Geometry: final body of the model. Coordinates: model frame, mm. A direction names the side the tool comes from. Give positions to 0.01 mm unless a question says otherwise; leave off trailing zeros. Write each loop counter-clockwise with the first axis right and the second up, starting at its lowest first coordinate (ties: lowest second). Pieces come first, ordered by that corner, then holes.
Q1. Draft query along Y for faces 6 (the face through (0, 31.828, 21)), 7 (the face through (-34, 13, -19.964)), 8 (the face through (34.03, 12.53, 21.44)). Return one class per face: pulls with the +Y half, pulls with the -Y half, needs draft (parallel to the pull), parting line crosses it, or undercut.
Q2. Cut plane D-D on y = 14.25. Return the cut outline in (x, z) (3 decimals), plus the area to 3 significant figures.
Q3. Line query: L1, parallel to Z at x = 30.5, y = 9.5; L2, parallel to Y at x = -23, z = -13; L3, parallel to Z at x = 23.5, y = 18. Output: solid intervals per line, ascending.
Q4. Pin query (flat end, axial travel): pin 1 (6.5 mm diameter, centred on y = 25, z = -16.5, fed in from +X) (3 decimals); pin 2 (6 mm diameter, centred on x = -25.5, y = 26, fed in from -Z); pin 3 (5 mm diameter, centred on x = -10.5, y = 24, fed in from -Z). Return the tip coordinate at first contact, or that it passes through.
Q5. Cut plane A-A on y = 22. Return the cut outline in (x, z) (1 decimal).
Q6. Cut plane B-B on z = 8. Return the cut outline in (x, y) (1 decimal).
Q7. Cut plane C-C on x = -3. Return the cut outline in (y, z).
Q8. Reachability of faces 1 (the face through (-4, 26.828, -15)), 2 (the face through (-1.495, 24.5, -15.2)), 3 (the face through (0, 24, 18.288)), 4 (the face through (-41, 19, -18.288)), 5 (the face through (0, 26, -8.032)) from +Z, -Z, +X, -X, +Y, -Y: full face, straight path, thin tool, end or side. Return the list, or none.
```python
from build123d import *

# Parameters (mm, degrees)
SKETCH1_W               = 36.575
SKETCH1_H               = 41.655
SKETCH1_W_2             = 28.575
SKETCH1_H_2             = 33.655
BOSS_EXTRUDE1_DEPTH     = 41.275
SKETCH2_W               = 36.575
SKETCH2_H               = 41.655
BOSS_EXTRUDE2_DEPTH     = 2
SKETCH4_W               = 86.55
SKETCH4_H               = 36.575
CUT_EXTRUDE2_DEPTH      = 37.655
SKETCH5_W               = 10.7752
SKETCH5_H               = 4
BOSS_EXTRUDE3_DEPTH     = 1.6764
SKETCH6_W               = 10.7752
SKETCH6_H               = 14.7752
SKETCH6_R               = 1.1
BOSS_EXTRUDE4_DEPTH     = 3
MIRROR3_COPY_1_SKETCH_W = 10.7752
MIRROR3_COPY_1_SKETCH_H = 4
MIRROR3_COPY_1_DEPTH    = 1.6764
MIRROR3_COPY_2_SKETCH_W = 10.7752
MIRROR3_COPY_2_SKETCH_H = 14.7752
MIRROR3_COPY_2_SKETCH_R = 1.1
MIRROR3_COPY_2_DEPTH    = 3
SKETCH7_W               = 4
SKETCH7_H               = 6
BOSS_EXTRUDE5_DEPTH     = 6
SKETCH8_R               = 0.381
CUT_EXTRUDE3_DEPTH      = 58.021122047
SKETCH9_W               = 41.02
SKETCH9_H               = 28.32
SKETCH9_W_2             = 33.02
SKETCH9_H_2             = 20.32
BOSS_EXTRUDE6_DEPTH     = 3
SKETCH10_W              = 41.02
SKETCH10_H              = 28.32
SKETCH10_W_2            = 37.02
SKETCH10_H_2            = 24.32
BOSS_EXTRUDE7_DEPTH     = 4
BOSS_EXTRUDE8_DEPTH     = 30
BOSS_EXTRUDE9_DEPTH     = 3.5
SKETCH13_W              = 55
SKETCH13_H              = 11
CUT_EXTRUDE4_DEPTH      = 3.175


with BuildPart() as part:
    # Sketch1 → Boss-Extrude1 (new, symmetric)
    with BuildSketch(Plane(origin=(0, 0, 0), x_dir=(0, 0, -1), z_dir=(1, 0, 0))):
        Rectangle(SKETCH1_W, SKETCH1_H)
        Rectangle(SKETCH1_W_2, SKETCH1_H_2, mode=Mode.SUBTRACT)
    extrude(amount=BOSS_EXTRUDE1_DEPTH, both=True)

    # Sketch2 → Boss-Extrude2 (add)
    with BuildSketch(Plane.ZY.offset(41.275)):
        Rectangle(SKETCH2_W, SKETCH2_H)
    boss_extrude2 = extrude(amount=BOSS_EXTRUDE2_DEPTH)

    # Mirror1: Boss-Extrude2 across plane
    add(boss_extrude2.mirror(Plane(origin=(0, 0, 0), x_dir=(0, 0, 1), z_dir=(1, 0, 0))))

    # Sketch4 → Cut-Extrude2 (cut)
    with BuildSketch(Plane.XZ.offset(20.8275)):
        Rectangle(SKETCH4_W, SKETCH4_H)
    extrude(amount=-CUT_EXTRUDE2_DEPTH, mode=Mode.SUBTRACT)

    # Sketch5 → Boss-Extrude3 (add)
    with BuildSketch(Plane(origin=(0, 0, -18.2875), x_dir=(-1, 0, 0), z_dir=(0, 0, -1))):
        with Locations((-33.8874, 18.8275)):
            Rectangle(SKETCH5_W, SKETCH5_H)
    boss_extrude3 = extrude(amount=BOSS_EXTRUDE3_DEPTH)

    # Sketch6 → Boss-Extrude4 (add)
    with BuildSketch(Plane(origin=(0, 0, -19.9639), x_dir=(-1, 0, 0), z_dir=(0, 0, -1))):
        with Locations((-33.8874, 13.4399)):
            Rectangle(SKETCH6_W, SKETCH6_H)
        with Locations((-33.8874, 11.4399)):
            Circle(SKETCH6_R, mode=Mode.SUBTRACT)
    boss_extrude4 = extrude(amount=BOSS_EXTRUDE4_DEPTH)

    # Mirror2: Boss-Extrude3, Boss-Extrude4 across plane
    add(boss_extrude3.mirror(Plane(origin=(0, 0, 0), x_dir=(0, 0, 1), z_dir=(1, 0, 0))))
    add(boss_extrude4.mirror(Plane(origin=(0, 0, 0), x_dir=(0, 0, 1), z_dir=(1, 0, 0))))

    # Mirror3: Boss-Extrude3, Boss-Extrude4 across plane
    add(boss_extrude3.mirror(Plane.XY))
    add(boss_extrude4.mirror(Plane.XY))

    # Mirror3 copy 1 sketch → Mirror3 copy 1 (add)
    with BuildSketch(Plane.XY.offset(18.2875)):
        with Locations((-33.8874, 18.8275)):
            Rectangle(MIRROR3_COPY_1_SKETCH_W, MIRROR3_COPY_1_SKETCH_H)
    extrude(amount=MIRROR3_COPY_1_DEPTH)

    # Mirror3 copy 2 sketch → Mirror3 copy 2 (add)
    with BuildSketch(Plane.XY.offset(19.9639)):
        with Locations((-33.8874, 13.4399)):
            Rectangle(MIRROR3_COPY_2_SKETCH_W, MIRROR3_COPY_2_SKETCH_H)
        with Locations((-33.8874, 11.4399)):
            Circle(MIRROR3_COPY_2_SKETCH_R, mode=Mode.SUBTRACT)
    extrude(amount=MIRROR3_COPY_2_DEPTH)

    # Sketch7 → Boss-Extrude5 (add)
    with BuildSketch(Plane(origin=(0, 20.8275, 0), x_dir=(1, 0, 0), z_dir=(0, 1, 0))):
        with Locations((-3.495, 15.2875)):
            Rectangle(SKETCH7_W, SKETCH7_H)
    extrude(amount=BOSS_EXTRUDE5_DEPTH)

    # Sketch8 → Cut-Extrude3 (cut, through all)
    with BuildSketch(Plane(origin=(-1.495, 0, 0), x_dir=(0, 0, -1), z_dir=(1, 0, 0))):
        with Locations((15.2875, 23.8275)):
            Circle(SKETCH8_R)
    extrude(amount=-CUT_EXTRUDE3_DEPTH, mode=Mode.SUBTRACT)

    # Sketch9 → Boss-Extrude6 (add)
    with BuildSketch(Plane(origin=(0, 20.8275, 0), x_dir=(1, 0, 0), z_dir=(0, 1, 0))):
        with Locations((0, -4.1275)):
            Rectangle(SKETCH9_W, SKETCH9_H)
        with Locations((0, -4.1275)):
            Rectangle(SKETCH9_W_2, SKETCH9_H_2, mode=Mode.SUBTRACT)
    extrude(amount=BOSS_EXTRUDE6_DEPTH)

    # Sketch10 → Boss-Extrude7 (add)
    with BuildSketch(Plane(origin=(0, 23.8275, 0), x_dir=(1, 0, 0), z_dir=(0, 1, 0))):
        with Locations((0, -4.1275)):
            Rectangle(SKETCH10_W, SKETCH10_H)
        with Locations((0, -4.1275)):
            Rectangle(SKETCH10_W_2, SKETCH10_H_2, mode=Mode.SUBTRACT)
    extrude(amount=BOSS_EXTRUDE7_DEPTH)

    # Sketch11 → Boss-Extrude8 (add, symmetric)
    with BuildSketch(Plane(origin=(0, 0, 0), x_dir=(0, 0, -1), z_dir=(1, 0, 0))):
        Polygon((-18.2875, 31.8275), (-23.2625, 31.8275), (-23.2625, 29.8275), (-20.0875, 29.8275), (-20.0875, 29.3275), (-18.2875, 29.3275), (-18.2875, 19.3275), (-20.0875, 19.3275), (-20.0875, 18.8275), (-23.2625, 18.8275), (-23.2625, 16.8275), (-18.2875, 16.8275), (-16.2875, 16.8275), (-16.2875, 27.8275), align=None)
    extrude(amount=BOSS_EXTRUDE8_DEPTH, both=True)

    # Sketch12 → Boss-Extrude9 (add)
    with BuildSketch(Plane.ZY.offset(30)):
        Polygon((23.2625, 29.8275), (23.2625, 18.8275), (18.2875, 18.8275), (18.2875, 29.3275), (20.0875, 29.3275), (20.0875, 29.8275), align=None)
    boss_extrude9 = extrude(amount=-BOSS_EXTRUDE9_DEPTH)

    # Mirror4: Boss-Extrude9 across plane
    add(boss_extrude9.mirror(Plane(origin=(0, 0, 0), x_dir=(0, 0, 1), z_dir=(1, 0, 0))))

    # Sketch13 → Cut-Extrude4 (cut)
    with BuildSketch(Plane.XY.offset(23.2625)):
        with Locations((0, 24.3275)):
            Rectangle(SKETCH13_W, SKETCH13_H)
    extrude(amount=-CUT_EXTRUDE4_DEPTH, mode=Mode.SUBTRACT)


solid = part.part
```
Data:
1. face 6: pulls with the +Y half
1. face 7: needs draft
1. face 8: undercut
2. outline: (-39.275, -22.964) - (-28.5, -22.964) - (-28.5, -19.964) - (-39.275, -19.964) - close; (-39.275, 19.964) - (-28.5, 19.964) - (-28.5, 22.964) - (-39.275, 22.964) - close; (28.5, -22.964) - (39.275, -22.964) - (39.275, -19.964) - (28.5, -19.964) - close; (28.5, 19.964) - (39.275, 19.964) - (39.275, 22.964) - (28.5, 22.964) - close
2. area: 129 mm2
3. L1: z = -22.96 to -19.96, 19.96 to 22.96
3. L2: y = 16.83 to 20.83
3. L3: z = -18.29 to 23.26
4. pin 1: stops at x = -1.495
4. pin 2: stops at z = 16.29
4. pin 3: stops at z = -10.03
5. outline: (-30, 16.3) - (-20.5, 16.3) - (-20.5, -10) - (20.5, -10) - (20.5, 16.3) - (30, 16.3) - (30, 23.3) - (27.5, 23.3) - (27.5, 20.1) - (26.5, 20.1) - (26.5, 18.3) - (-26.5, 18.3) - (-26.5, 20.1) - (-27.5, 20.1) - (-27.5, 23.3) - (-30, 23.3) - close; (-5.5, -18.3) - (-1.5, -18.3) - (-1.5, -12.3) - (-5.5, -12.3) - close; hole (-16.5, -6) - (16.5, -6) - (16.5, 14.3) - (-16.5, 14.3) - close
6. outline: (-43.3, 16.8) - (43.3, 16.8) - (43.3, 20.8) - (20.5, 20.8) - (20.5, 27.8) - (18.5, 27.8) - (18.5, 23.8) - (16.5, 23.8) - (16.5, 20.8) - (-16.5, 20.8) - (-16.5, 23.8) - (-18.5, 23.8) - (-18.5, 27.8) - (-20.5, 27.8) - (-20.5, 20.8) - (-43.3, 20.8) - close
7. outline: (16.83, -18.29) - (26.83, -18.29) - (26.83, -12.29) - (20.83, -12.29) - (20.83, -10.03) - (27.83, -10.03) - (27.83, -8.03) - (23.83, -8.03) - (23.83, -6.03) - (20.83, -6.03) - (20.83, 14.29) - (23.83, 14.29) - (23.83, 16.29) - (27.83, 16.29) - (31.83, 18.29) - (31.83, 23.26) - (29.83, 23.26) - (29.83, 20.09) - (29.33, 20.09) - (29.33, 18.29) - (19.33, 18.29) - (19.33, 20.09) - (18.83, 20.09) - (18.83, 23.26) - (16.83, 23.26) - close; hole circle Ø0.76 at (23.83, -15.29)
8. face 1: -Z, +X, -X, +Y
8. face 2: -Z, +X, +Y
8. face 3: +Z
8. face 4: -Z, -X, +Y, -Y
8. face 5: +Y
